Can you work these out from the model? Positions are in its coordinate system, mm. A direction names the side the tool comes from. Coordinates: 2 decimals unless noted, no trailing zeros. Order: outer loops, then holes, each group sorted by start corner. A loop starts at its lowest first (then second) coordinate and runs counter-clockwise, first axis right, second up.
```python
from build123d import *

# Parameters (mm, degrees)
SKETCH1_R           = 13.5
SKETCH1_R_2         = 4.5
BOSS_EXTRUDE1_DEPTH = 0.4
SKETCH2_R           = 3
BOSS_EXTRUDE3_DEPTH = 1.9


with BuildPart() as part:
    # Sketch1 → Boss-Extrude1 (new, symmetric)
    with BuildSketch(Plane(origin=(0, 0, 0), x_dir=(1, 0, 0), z_dir=(0, 1, 0))):
        with Locations(Location((0, 0, 0), (0, 0, 270))):
            Circle(SKETCH1_R)
        with Locations(Location((0, 0, 0), (0, 0, 270))):
            Circle(SKETCH1_R_2, mode=Mode.SUBTRACT)
    extrude(amount=BOSS_EXTRUDE1_DEPTH, both=True)

    # Sketch2 → Boss-Extrude3 (add)
    with BuildSketch(Plane(origin=(0, 0, 0), x_dir=(1, 0, 0), z_dir=(0, 1, 0))):
        with Locations(Location((0, 9, 0), (0, 0, 270))):
            Circle(SKETCH2_R)
        with Locations(Location((9, 0, 0), (0, 0, 270))):
            Circle(SKETCH2_R)
        with Locations(Location((-9, 0, 0), (0, 0, 270))):
            Circle(SKETCH2_R)
        with Locations(Location((0, -9, 0), (0, 0, 270))):
            Circle(SKETCH2_R)
    extrude(amount=-BOSS_EXTRUDE3_DEPTH)


solid = part.part
```
1. On a 3-axis mill with a long thin cutter (end or side, diameter ignored), from which of +Z, -Z, +X, -X, +Y, -Y can I reach the whole of each face in a straight line? I mean faces 4 (the cylindrical face through (0, -1, -12)), 5 (the flat face through (-9, -1.9, 0)). Say none if no direction works.
Completed:
face 4: -Y
face 5: +Z, -Z, +X, -X, -Y
2. Imagine slicing it at D-D on y = -0.05. Please give me the cut outline in (x, z), then the cut area to 3 significant figures.
Completed:
outline: circle Ø27 at (0, 0); hole circle Ø9 at (0, 0)
area: 509 mm2
3. Imagine slicing it at B-B on x = 0. Please give me the cut outline in (y, z).
Completed:
outline: (-1.9, -12) - (-0.4, -12) - (-0.4, -13.5) - (0.4, -13.5) - (0.4, -4.5) - (-0.4, -4.5) - (-0.4, -6) - (-1.9, -6) - close; (-1.9, 6) - (-0.4, 6) - (-0.4, 4.5) - (0.4, 4.5) - (0.4, 13.5) - (-0.4, 13.5) - (-0.4, 12) - (-1.9, 12) - close
4. Imagine slicing it at C-C on y = -1.5. Please give me the cut outline in (x, z).
Completed:
outline: circle Ø6 at (-9, 0); circle Ø6 at (0, -9); circle Ø6 at (0, 9); circle Ø6 at (9, 0)
5. Imagine slicing it at A-A on z = 0. Please give me the cut outline in (x, y).
Completed:
outline: (-13.5, -0.4) - (-12, -0.4) - (-12, -1.9) - (-6, -1.9) - (-6, -0.4) - (-4.5, -0.4) - (-4.5, 0.4) - (-13.5, 0.4) - close; (4.5, -0.4) - (6, -0.4) - (6, -1.9) - (12, -1.9) - (12, -0.4) - (13.5, -0.4) - (13.5, 0.4) - (4.5, 0.4) - close
6. I'm going to push a flat-ended pin straight in: pin 1 (2 mm diameter, centred on x = -5, z = 6, fed in from -Y). Where does the tip first touch, or does it pass through?
Completed:
pin 1: stops at y = -0.4
7. Please list where these lines run through material, in increasing order: probe 1 along X at (y, z) = (0, 0); probe 2 along Y at (x, z) = (-8, 5); probe 3 along X at (y, z) = (0.05, 3.25).
Completed:
probe 1: x = -13.5 to -4.5, 4.5 to 13.5
probe 2: y = -0.4 to 0.4
probe 3: x = -13.1 to -3.11, 3.11 to 13.1
8. Thinking about a two-plate mould opening in X: for faces 1 (the cylindrical face through (-6, -1, 0)), 2 (the cylindrical face through (-13.18, 0.01, -2.93)), 3 (the flat face through (0, -1.9, 9)), which applies, pulls with the +X half, pulls with the -X half, needs draft (parallel to the pull), parting line crosses it, or undercut?
Completed:
face 1: undercut
face 2: parting line crosses it
face 3: needs draft
